from build123d import *

# Parameters (mm, degrees)
BOSS_EXTRUDE1_DEPTH = 6.35
SKETCH4_W           = 4.7625
SKETCH4_H           = 9.525
SKETCH4_W_2         = 9.525
SKETCH4_H_2         = 3.175
CUT_EXTRUDE1_DEPTH  = 6.35
SKETCH6_W           = 38.1
SKETCH6_H           = 6.35
BOSS_EXTRUDE3_DEPTH = 6.35


with BuildPart() as part:
    # Sketch2 → Boss-Extrude1 (new body)
    with BuildSketch(Plane(origin=(0, 0, 0), x_dir=(0, 0, -1), z_dir=(1, 0, 0))):
        Polygon((0, 127), (0, 0), (12.7, 0), (12.7, 114.3), (15.875, 114.3), (50.8, 114.3), (50.8, 0), (63.5, 0), (63.5, 114.3), (63.5, 127), (49.2125, 127), (49.2125, 133.35), (36.5125, 133.35), (36.5125, 127), (23.8125, 127), (23.8125, 133.35), (11.1125, 133.35), (11.1125, 127), align=None)
        Polygon((4.35, 6.35), (4.35, 120.65), (6.35, 120.65), (8.35, 120.65), (8.35, 6.35), align=None, mode=Mode.SUBTRACT)
        Polygon((59.15, 120.65), (59.15, 114.3), (59.15, 6.35), (55.15, 6.35), (55.15, 114.3), (55.15, 120.65), (57.15, 120.65), align=None, mode=Mode.SUBTRACT)
    extrude(amount=BOSS_EXTRUDE1_DEPTH)

    # Sketch4 → Cut-Extrude1 (cut)
    with BuildSketch(Plane.ZY):
        with Locations((-30.1625, 122.2375)):
            Rectangle(SKETCH4_W, SKETCH4_H)
        with Locations((-30.1625, 122.2375)):
            Rectangle(SKETCH4_W_2, SKETCH4_H_2)
    extrude(amount=-CUT_EXTRUDE1_DEPTH, mode=Mode.SUBTRACT)

    # Sketch6 → Boss-Extrude3 (add)
    with BuildSketch(Plane(origin=(6.35, 0, 0), x_dir=(0, 0, -1), z_dir=(1, 0, 0))):
        with Locations((31.75, 3.175)):
            Rectangle(SKETCH6_W, SKETCH6_H)
    extrude(amount=-BOSS_EXTRUDE3_DEPTH)


solid = part.part
Build history of the part. All positions in model axes, mm. A direction names the side the tool comes from. Round coordinates to 2 decimals unless told otherwise and drop trailing zeros. Write each loop counter-clockwise with the first axis right and the second up, starting at its lowest first coordinate (ties: lowest second). Pieces come first, ordered by that corner, then holes. Notation, with made-up numbers: M -7,-19.75 L 4,-19.75 A24 ccw 4,18.25 Z; hole C 65.5,-10.5 d6. An arc over 180 degrees is marked long. Answer as a JSON object with one key per item and string values. Group by question number.
(1) Drill centre lines: L1, parallel to Z at x = 2.5, y = 93; L2, parallel to Y at x = 2.5, z = -26.5 (3 decimals); L3, parallel to Y at x = 3.25, z = -19.5. Where is each one in solid material? Low to high.
(2) Cut at C-C (x = 2.25). Give the number of separate pieces and of enclosed holes in the cut face, and give its area (3 significant figures).
(3) Cut at B-B (y = 35). Give the cut face in (x, z), and give its area (3 significant figures).
(4) Cut at A-A (z = -20). Give the cut face in (x, y), and give its area (3 significant figures).
(5) Which spindle directions (+Z, -Z, +X, -X, +Y, -Y) get a long thin tool onto all of the face, cutting with end or side? Do faces 5 (the flat face through (3, 125, -27.781)), 6 (the flat face through (3, 6.35, -31)), 7 (the flat face through (3, 130, -11.112)), 8 (the flat face through (6.35, 68, -10)), 9 (the flat face through (3, 127, -56)). Say none if no direction does.
(6) Flat gauge pins, fed straight in: pin 1 (1.9 mm diameter, centred on x = 3.5, y = 130, fed in from -Z); pin 2 (1.2 mm diameter, centred on x = 2, z = -26.5, fed in from +Y); pin 3 (10 mm diameter, centred on y = 56.5, z = -45, fed in from -X). Where does each tip first touch, or does it go through?
(7) Cut at D-D (z = -52). Give the cut face in (x, y).
(8) Mould opens along Z. For faces 1 (the flat face through (3, 0, -31)), 2 (the flat face through (3, 130, -49.212)), 3 (the flat face through (3, 120.65, -6)), 4 (the flat face through (3, 114.3, -31)) say: pulls with the +Z half, pulls with the -Z half, needs draft (parallel to the pull), parting line crosses it, or undercut.
Responses:
{
 "1": {"L1": "z = -63.5 to -59.15, -55.15 to -50.8, -12.7 to -8.35, -4.35 to 0", "L2": "y = 0 to 6.35, 114.3 to 120.65, 123.825 to 127", "L3": "y = 0 to 6.35, 114.3 to 133.35"},
 "2": {"separate pieces": "1", "enclosed holes": "3", "area": "3,140 mm2"},
 "3": {"outline": "M 0,-63.5 L 6.35,-63.5 L 6.35,-59.15 L 0,-59.15 Z; M 0,-55.15 L 6.35,-55.15 L 6.35,-50.8 L 0,-50.8 Z; M 0,-12.7 L 6.35,-12.7 L 6.35,-8.35 L 0,-8.35 Z; M 0,-4.35 L 6.35,-4.35 L 6.35,0 L 0,0 Z", "area": "110 mm2"},
 "4": {"outline": "M 0,0 L 6.35,0 L 6.35,6.35 L 0,6.35 Z; M 0,114.3 L 6.35,114.3 L 6.35,133.35 L 0,133.35 Z", "area": "161 mm2"},
 "5": {"face 5": "+X, -X, +Y", "face 6": "+X, -X", "face 7": "+Z, +X, -X, +Y", "face 8": "+Z, -Z, +X, +Y, -Y", "face 9": "-Z, +X, -X, +Y"},
 "6": {"pin 1": "stops at z = -49.21", "pin 2": "stops at y = 127", "pin 3": "passes through"},
 "7": {"outline": "M 0,0 L 6.35,0 L 6.35,127 L 0,127 Z"},
 "8": {"face 1": "needs draft", "face 2": "pulls with the -Z half", "face 3": "undercut", "face 4": "undercut"}
}
